Check sheet for the drawn part. Datum: minimum x, y, z corner. Units: mm. A direction names the side the tool comes from. Round coordinates to 2 decimals unless told otherwise and drop trailing zeros. Loops run counter-clockwise (first coordinate to the right, second up) from the corner with the lowest first, then second, coordinate; pieces in that order, holes last. Notation, with made-up numbers: (22.5, -35.5) -> (43.5, -35.5) arc R13 cw to (43.5, -28.5) -> close; hole circle Ø2 at (12.5, 28). An arc over 180 degrees is marked (long way). Return JSON: item names as keys, results as strings.
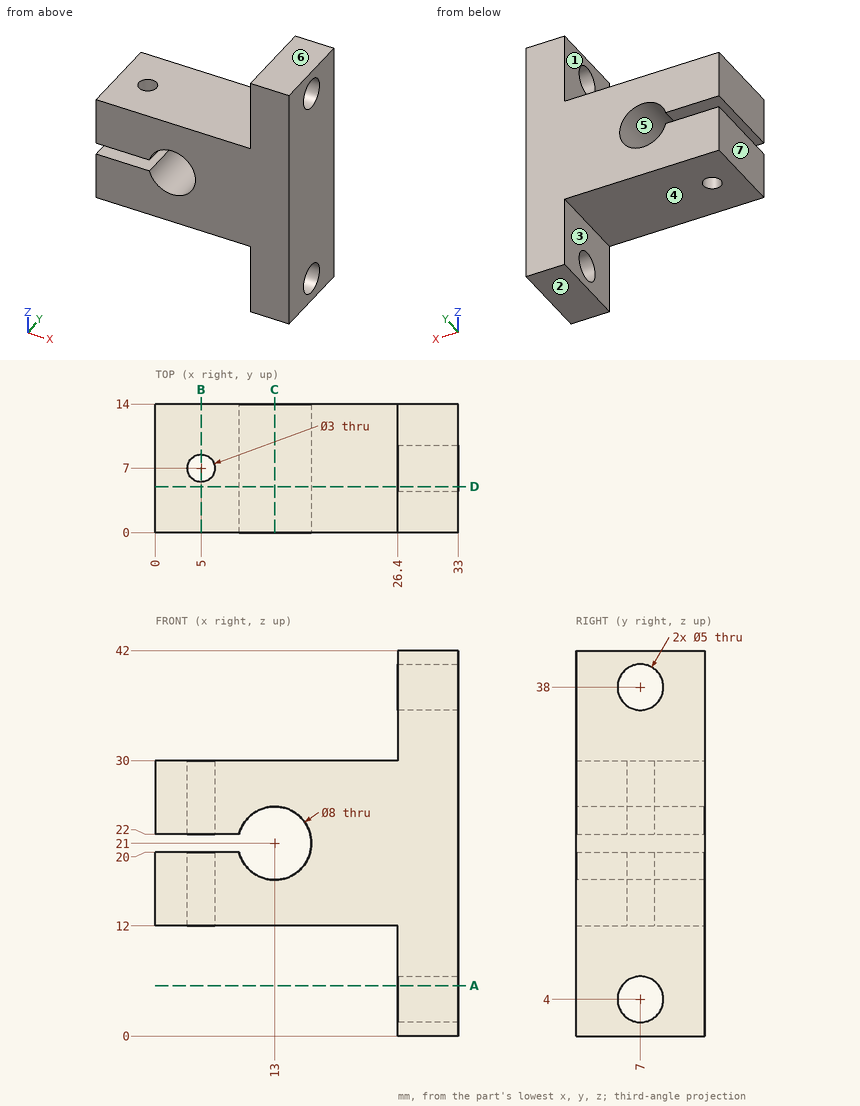
Q1. Section check A-A (z = 5.5). Record the boundary of the cut face in (x, y).
Results list:
{"outline": "(26.4, 0) -> (33, 0) -> (33, 5) -> (26.4, 5) -> close; (26.4, 9) -> (33, 9) -> (33, 14) -> (26.4, 14) -> close"}
Q2. Section check B-B (x = 5). Record the boundary of the cut face in (y, z), then the cut area to 3 significant figures.
Results list:
{"outline": "(0, 12) -> (5.5, 12) -> (5.5, 20) -> (0, 20) -> close; (0, 22) -> (5.5, 22) -> (5.5, 30) -> (0, 30) -> close; (8.5, 12) -> (14, 12) -> (14, 20) -> (8.5, 20) -> close; (8.5, 22) -> (14, 22) -> (14, 30) -> (8.5, 30) -> close", "area": "176 mm^2"}
Q3. Tool access check on the marked faces 1, 2 and 3. Record the directions out of +Z, -Z, +X, -X, +Y, -Y that give a thin tool (end or side, any length) a straight path to the whole face; none if there is none.
Results list:
{"face 1": "+Z, -X, +Y, -Y", "face 2": "-Z, +X, -X, +Y, -Y", "face 3": "-Z, -X, +Y, -Y"}
Q4. Section check D-D (y = 5). Record the boundary of the cut face in (x, z).
Results list:
{"outline": "(0, 12) -> (26.4, 12) -> (26.4, 5.5) -> (33, 5.5) -> (33, 36.5) -> (26.4, 36.5) -> (26.4, 30) -> (0, 30) -> (0, 22) -> (9.13, 22) arc R4 cw (long way) to (9.13, 20) -> (0, 20) -> close; (26.4, 0) -> (33, 0) -> (33, 2.5) -> (26.4, 2.5) -> close; (26.4, 39.5) -> (33, 39.5) -> (33, 42) -> (26.4, 42) -> close"}
Q5. Draft check along Z on the marked faces 4, 5, 6 and 7. Enter one of: released by +Z, released by -Z, zero draft, split by the parting line, or undercut.
Results list:
{"face 4": "released by -Z", "face 5": "undercut", "face 6": "released by +Z", "face 7": "zero draft"}
Q6. Material ranges on line 1 (Z direction, x = 13, y = 4); line 2 (Y direction, x = 5, z = 25); line 3 (Z direction, x = 3, y = 4), recorded low to high.
Results list:
{"line 1": "12 to 17, 25 to 30", "line 2": "0 to 5.5, 8.5 to 14", "line 3": "12 to 20, 22 to 30"}
Q7. Go/stop test with flat-tipped pins: pin 1 (1 mm diameter, centred on x = 7, y = 12.5, fed in from -Z); pin 2 (4 mm diameter, centred on y = 5, z = 8, fed in from -X); pin 3 (7 mm diameter, centred on x = 7.5, y = 8.5, fed in from +Z); pin 4 (1.8 mm diameter, centred on x = 5, y = 7, fed in from -Z). Record where each tip stops, or that it passes through.
Results list:
{"pin 1": "z = 12", "pin 2": "x = 26.4", "pin 3": "z = 30", "pin 4": "through"}
Q8. Section check C-C (x = 13). Record the boundary of the cut face in (y, z), then the cut area to 3 significant figures.
Results list:
{"outline": "(0, 12) -> (14, 12) -> (14, 17) -> (0, 17) -> close; (0, 25) -> (14, 25) -> (14, 30) -> (0, 30) -> close", "area": "140 mm^2"}
